Part model, mm, in its own coordinate system. A direction names the side the tool comes from. Round coordinates to 2 decimals unless told otherwise and drop trailing zeros. Write each loop counter-clockwise with the first axis right and the second up, starting at its lowest first coordinate (ties: lowest second). Pieces come first, ordered by that corner, then holes.
```python
from build123d import *

# Parameters (mm, degrees)
EXTRUDE_1_DEPTH = 1.5
EXTRUDE_2_DEPTH = 3


with BuildPart() as part:
    # 草圖1 → 擠出1 (new body)
    with BuildSketch(Plane.XY):
        Polygon((-16, 0), (0, 16), (0, 111), (-16, 111), (-16, 97.073509127), (-98.206395117, 0), align=None)
    extrude(amount=EXTRUDE_1_DEPTH)

    # 草圖2 → 擠出2 (add)
    with BuildSketch(Plane.XY):
        Polygon((-110, 0), (-98.206395117, 0), (-16, 97.073509127), (-16, 111), align=None)
    extrude(amount=EXTRUDE_2_DEPTH)


with BuildPart() as body_2:
    # 鏡射1: mirrored copy
    add(part.part.mirror(Plane(origin=(-44.219505569, 22.2, 0), x_dir=(1, 0, 0), z_dir=(0, 0, 1))))


solid = body_2.part
```
Q1. Wall check: L1, parallel to Z at x = -61, y = 14.5; L2, parallel to Y at x = -31, z = -2.3; L3, parallel to X at y = 68, z = -1.8. Give the ranges that are in metal, low to high.
Values follow:
L1: z = -1.5 to 0
L2: y = 79.36 to 93.29
L3: x = -52.41 to -40.62
Q2. Cut at A-A on z = -0.7. Write the cut outline in (x, y).
Values follow:
outline: (-110, 0) - (-16, 0) - (0, 16) - (0, 111) - (-16, 111) - close
Q3. Drop flat-ended pins along their axis: pin 1 (12 mm diameter, centred on x = -58.5, y = 16, fed in from -Z); pin 2 (1.2 mm diameter, centred on y = 106.5, z = -2.5, fed in from +X). Give the stop position or say it passes through.
Values follow:
pin 1: stops at z = -1.5
pin 2: stops at x = -16
Q4. Cut at C-C on y = 90. Write the cut outline in (x, z).
Values follow:
outline: (-33.78, -3) - (-21.99, -3) - (-21.99, -1.5) - (0, -1.5) - (0, 0) - (-33.78, 0) - close
Q5. Which spindle directions (+Z, -Z, +X, -X, +Y, -Y) get a long thin tool onto all of the face, cutting with end or side? Do faces 1 (the flat face through (-57.679, 47.857, -2.24)), 2 (the flat face through (-60, 52, -3)). Say none if no direction does.
Values follow:
face 1: -Z, +X, -Y
face 2: -Z, +X, -X, +Y, -Y
Q6. Cut at B-B on x = -64.5. Write the cut outline in (y, z).
Values follow:
outline: (0, -1.5) - (39.8, -1.5) - (39.8, -3) - (53.73, -3) - (53.73, 0) - (0, 0) - close
Q7. Cut at D-D on x = -100.5. Write the cut outline in (y, z), plus the area to 3 significant figures.
Values follow:
outline: (0, -3) - (11.22, -3) - (11.22, 0) - (0, 0) - close
area: 33.7 mm2
